```python
from build123d import *

# Parameters (mm, degrees)
BOSS_EXTRUDE1_DEPTH = 4
BOSS_EXTRUDE2_START = 4
SKETCH1_3_W         = 102.8
SKETCH1_3_H         = 62.8
BOSS_EXTRUDE2_DEPTH = 2
SKETCH2_R           = 1.5
CUT_EXTRUDE1_DEPTH  = 66.467549213
SKETCH2_3_R         = 3
CUT_EXTRUDE2_DEPTH  = 2


with BuildPart() as part:
    # Sketch1 → Boss-Extrude1 (new body)
    with BuildSketch(Plane(origin=(0, 0, 0), x_dir=(1, 0, 0), z_dir=(0, 1, 0))):
        with BuildLine():
            Line((-52, -35), (52, -35))
            ThreePointArc((52, -35), (54.121320344, -34.121320344), (55, -32))
            Line((55, -32), (55, 32))
            ThreePointArc((55, 32), (54.121320344, 34.121320344), (52, 35))
            Line((52, 35), (-52, 35))
            ThreePointArc((-52, 35), (-54.121320344, 34.121320344), (-55, 32))
            Line((-55, 32), (-55, -32))
            ThreePointArc((-55, -32), (-54.121320344, -34.121320344), (-52, -35))
        make_face()
    extrude(amount=BOSS_EXTRUDE1_DEPTH)

    # Sketch1<3> → Boss-Extrude2 (add)
    with BuildSketch(Plane(origin=(0, 0, 0), x_dir=(1, 0, 0), z_dir=(0, 1, 0)).offset(BOSS_EXTRUDE2_START)):
        with BuildLine():
            Line((-53.4, -32), (-53.4, 32))
            ThreePointArc((-53.4, 32), (-52.989949494, 32.989949494), (-52, 33.4))
            Line((-52, 33.4), (52, 33.4))
            ThreePointArc((52, 33.4), (52.989949494, 32.989949494), (53.4, 32))
            Line((53.4, 32), (53.4, -32))
            ThreePointArc((53.4, -32), (52.989949494, -32.989949494), (52, -33.4))
            Line((52, -33.4), (-52, -33.4))
            ThreePointArc((-52, -33.4), (-52.989949494, -32.989949494), (-53.4, -32))
        make_face()
        Rectangle(SKETCH1_3_W, SKETCH1_3_H, mode=Mode.SUBTRACT)
    extrude(amount=BOSS_EXTRUDE2_DEPTH)

    # Sketch2 → Cut-Extrude1 (cut, through all)
    with BuildSketch(Plane.XZ):
        with Locations(Location((-45.5, 27.5, 0), (0, 0, 270))):
            Circle(SKETCH2_R)
        with Locations(Location((45.5, 27.5, 0), (0, 0, 270))):
            Circle(SKETCH2_R)
        with Locations(Location((45.5, -27.5, 0), (0, 0, 270))):
            Circle(SKETCH2_R)
        with Locations(Location((-45.5, -27.5, 0), (0, 0, 270))):
            Circle(SKETCH2_R)
    extrude(amount=-CUT_EXTRUDE1_DEPTH, mode=Mode.SUBTRACT)

    # Sketch2<3> → Cut-Extrude2 (cut)
    with BuildSketch(Plane.XZ):
        with Locations(Location((-45.5, 27.5, 0), (0, 0, 270))):
            Circle(SKETCH2_3_R)
        with Locations(Location((45.5, 27.5, 0), (0, 0, 270))):
            Circle(SKETCH2_3_R)
        with Locations(Location((45.5, -27.5, 0), (0, 0, 270))):
            Circle(SKETCH2_3_R)
        with Locations(Location((-45.5, -27.5, 0), (0, 0, 270))):
            Circle(SKETCH2_3_R)
    extrude(amount=-CUT_EXTRUDE2_DEPTH, mode=Mode.SUBTRACT)


solid = part.part
```
Work out the finished part from the listing and answer in its coordinate system (mm). A direction names the side the tool comes from. Give positions to 0.01 mm unless a question says otherwise; leave off trailing zeros. Loops run counter-clockwise (first coordinate to the right, second up) from the corner with the lowest first, then second, coordinate; pieces in that order, holes last. Notation, with made-up numbers: (21, 85.25) - (67, 85.25) arc R6 cw to (67, 91.25) - close; hole circle Ø8 at (-36, 28). An arc over 180 degrees is marked (long way). Use CSV: the item, a comma, the result in double quotes. Start each with the question number.
(1) Find the intervals of material crossed by L1, parallel to X at y = 1.55, z = 27.5; L2, parallel to Z at x = 2.5, y = 4.55; L3, parallel to X at y = 4.1, z = -23, in increasing order.
(2) Determine the mould class of faces 1 (the face through (16, 6, -32)), 2 (the face through (-1, 2, 35)), 3 (the face through (-1, 5, -33.4)), 4 (the face through (-1, 5, 31.4)) for opening direction Z: released by +Z, released by -Z, zero draft, split by the parting line, or undercut.
(3) A tool of negligible diameter and unlimited length cuts with its end or side. For faces 5 (the face through (-1, 5, -31.4)), 6 (the face through (-55, 2, 0)), 7 (the face through (-53.4, 5, 0)), 8 (the face through (-43.47, 0.99, -25.29)), 9 (the face through (55, 2, 0)), from which of +Z, -Z, +X, -X, +Y, -Y can it reach the whole face along a straight path? Write none if from no direction.
(4) Find section C-C, the plane x = -34.5. Determine the outline of the cut face in (y, z).
(5) Each of these flat-tipped pins is pushed along its axis until it touches: pin 1 (5.5 mm diameter, centred on x = 45.5, z = 27.5, fed in from +Y); pin 2 (5 mm diameter, centred on x = -46.5, z = -28, fed in from -Y); pin 3 (1 mm diameter, centred on x = 21, y = 5, fed in from +Z); pin 4 (1.8 mm diameter, centred on x = 46, z = 27.5, fed in from -Y) (1 decimal). Where does it stop, or does it pass through?
(6) Find section A-A, the plane x = -45.5. Determine the outline of the cut face in (y, z), plus the area to 3 significant figures.
(7) Find section B-B, the plane z = 27.5. Determine the outline of the cut face in (x, y), plus the area to 3 significant figures.
(8) Find section D-D, the plane z = 3. Determine the outline of the cut face in (x, y), plus the area to 3 significant figures.
Results found:
1,L1,"-55 to -48.5, -42.5 to 42.5, 48.5 to 55"
1,L2,"-33.4 to -31.4, 31.4 to 33.4"
1,L3,"-53.4 to -51.4, 51.4 to 53.4"
2,face 1,"zero draft"
2,face 2,"released by +Z"
2,face 3,"released by -Z"
2,face 4,"undercut"
3,face 5,"+Y"
3,face 6,"+Z, -Z, -X, +Y, -Y"
3,face 7,"+Z, -Z, -X, +Y"
3,face 8,"-Y"
3,face 9,"+Z, -Z, +X, +Y, -Y"
4,outline,"(0, -35) - (4, -35) - (4, -33.4) - (6, -33.4) - (6, -31.4) - (4, -31.4) - (4, 31.4) - (6, 31.4) - (6, 33.4) - (4, 33.4) - (4, 35) - (0, 35) - close"
5,pin 1,"y = 4"
5,pin 2,"y = 0"
5,pin 3,"z = 33.4"
5,pin 4,"through"
6,outline,"(0, -35) - (4, -35) - (4, -33.4) - (6, -33.4) - (6, -31.4) - (4, -31.4) - (4, -29) - (2, -29) - (2, -30.5) - (0, -30.5) - close; (0, -24.5) - (2, -24.5) - (2, -26) - (4, -26) - (4, 26) - (2, 26) - (2, 24.5) - (0, 24.5) - close; (0, 30.5) - (2, 30.5) - (2, 29) - (4, 29) - (4, 31.4) - (6, 31.4) - (6, 33.4) - (4, 33.4) - (4, 35) - (0, 35) - close"
6,area,"252 mm^2"
7,outline,"(-55, 0) - (-48.5, 0) - (-48.5, 2) - (-47, 2) - (-47, 4) - (-51.4, 4) - (-51.4, 6) - (-53.4, 6) - (-53.4, 4) - (-55, 4) - close; (-44, 2) - (-42.5, 2) - (-42.5, 0) - (42.5, 0) - (42.5, 2) - (44, 2) - (44, 4) - (-44, 4) - close; (47, 2) - (48.5, 2) - (48.5, 0) - (55, 0) - (55, 4) - (53.4, 4) - (53.4, 6) - (51.4, 6) - (51.4, 4) - (47, 4) - close"
7,area,"412 mm^2"
8,outline,"(-55, 0) - (55, 0) - (55, 4) - (53.4, 4) - (53.4, 6) - (51.4, 6) - (51.4, 4) - (-51.4, 4) - (-51.4, 6) - (-53.4, 6) - (-53.4, 4) - (-55, 4) - close"
8,area,"448 mm^2"
